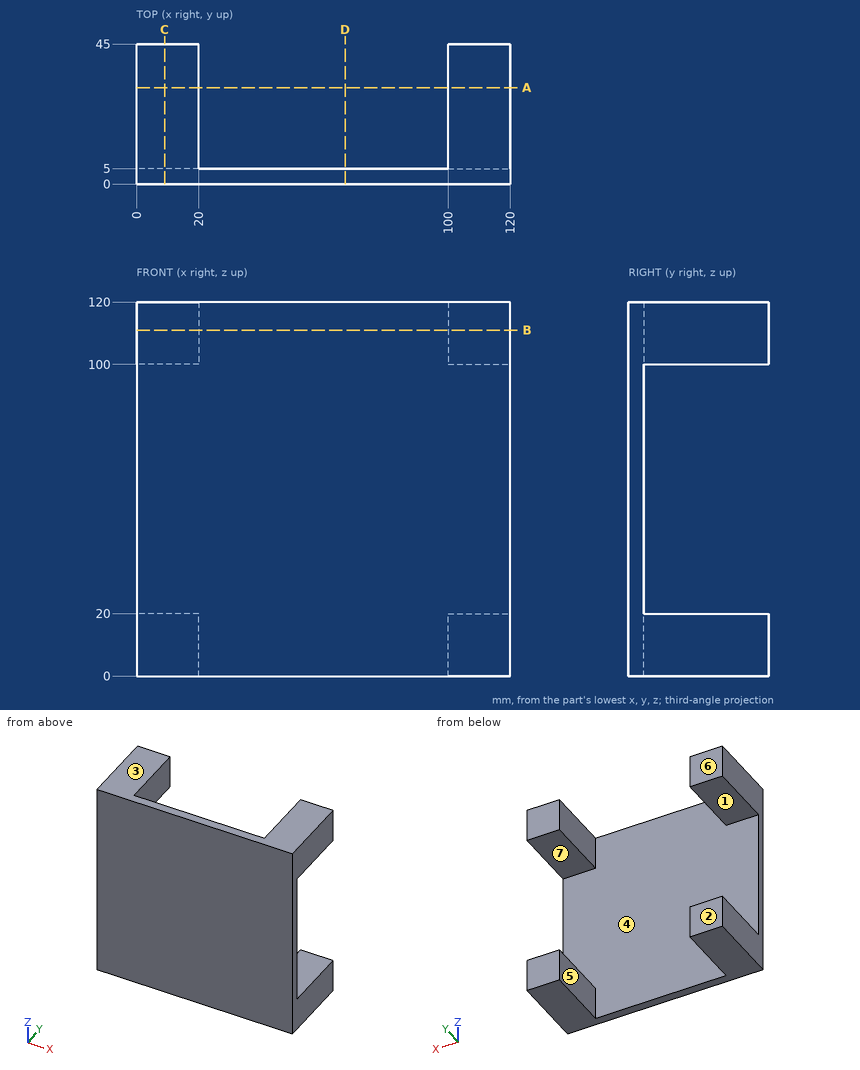
Verification items for this drawing (mm, ordinates from the low corner). A direction names the side the tool comes from. Round coordinates to 2 decimals unless told otherwise and drop trailing zeros. Loops run counter-clockwise (first coordinate to the right, second up) from the corner with the lowest first, then second, coordinate; pieces in that order, holes last. Notation, with made-up numbers: M 73.25,-38.5 L 84.25,-38.5 A18 cw 84.25,-11.5 Z; hole C 23.25,72 d2. An arc over 180 degrees is marked long. Answer as a JSON object with one key per item and string values.
1. Scan lines: line 1 (X direction, y = 34, z = 5.5); line 2 (Y direction, x = 81.5, z = 10). Record each from-to range of solid material in increasing order.
Reply:
{"line 1": "x = 0 to 20, 100 to 120", "line 2": "y = 0 to 5"}
2. Section check A-A (y = 31). Record the boundary of the cut face in (x, z).
Reply:
{"outline": "M 0,0 L 20,0 L 20,20 L 0,20 Z; M 0,100 L 20,100 L 20,120 L 0,120 Z; M 100,0 L 120,0 L 120,20 L 100,20 Z; M 100,100 L 120,100 L 120,120 L 100,120 Z"}
3. Section check C-C (x = 9). Record the boundary of the cut face in (y, z).
Reply:
{"outline": "M 0,0 L 45,0 L 45,20 L 5,20 L 5,100 L 45,100 L 45,120 L 0,120 Z"}
4. Access from +Z, -Z, +X, -X, +Y, -Y to the whole of each face (thin tool, end or side, straight path). Record for the marked faces 5, 6 and 7.
Reply:
{"face 5": "+Z, -Z, +Y", "face 6": "+Z, -Z, +X, -X, +Y", "face 7": "+X, -X, +Y"}
5. Section check B-B (z = 111). Record the boundary of the cut face in (x, y), plus the area to 3 significant figures.
Reply:
{"outline": "M 0,0 L 120,0 L 120,45 L 100,45 L 100,5 L 20,5 L 20,45 L 0,45 Z", "area": "2,200 mm²"}
6. Gauge pin test, flat end, axial feed: P1, Ø4, axis at x = 28.5, z = 64, coming from the +Y side. Record the tip position at first contact, or that the pin passes through.
Reply:
{"P1": "stops at y = 5"}
7. Mould release check, pull along Z, two halves, no side actions. Record for the marked faces 1, 2, 3 and 4: pulls with the +Z half, pulls with the -Z half, needs draft (parallel to the pull), parting line crosses it, or undercut.
Reply:
{"face 1": "undercut", "face 2": "needs draft", "face 3": "pulls with the +Z half", "face 4": "undercut"}
8. Section check D-D (x = 67). Record the boundary of the cut face in (y, z), plus the area to 3 significant figures.
Reply:
{"outline": "M 0,0 L 5,0 L 5,120 L 0,120 Z", "area": "600 mm²"}
